Design review of the part built by this model. Coordinates are the model's own, in mm. Round coordinates to 2 decimals unless told otherwise and drop trailing zeros. Loops run counter-clockwise (first coordinate to the right, second up) from the corner with the lowest first, then second, coordinate; pieces in that order, holes last. Notation, with made-up numbers: (-32, -8.5) -> (-28, -8.5) arc R8 cw to (-28, -1.5) -> close; hole circle Ø11 at (89, 69). An arc over 180 degrees is marked (long way). Use a Markdown table: item, result. Add a question column.
from build123d import *

# Parameters (mm, degrees)
SKETCH1_R           = 3.9751
SKETCH1_R_2         = 6.35
BOSS_EXTRUDE1_DEPTH = 3.175


with BuildPart() as part:
    # Sketch1 → Boss-Extrude1 (new body)
    with BuildSketch(Plane.XY):
        with BuildLine():
            Line((-25.4, 88.9), (25.4, 88.9))
            Line((25.4, 88.9), (50.793088675, 18.258224664))
            ThreePointArc((50.793088675, 18.258224664), (0, -53.975), (-50.793088675, 18.258224664))
            Line((-50.793088675, 18.258224664), (-25.4, 88.9))
        make_face()
        with Locations((14.2875, 79.375)):
            Circle(SKETCH1_R, mode=Mode.SUBTRACT)
        with Locations(Location((-14.2875, 79.375, 0), (0, 0, 180))):
            Circle(SKETCH1_R, mode=Mode.SUBTRACT)
        Circle(SKETCH1_R_2, mode=Mode.SUBTRACT)
    extrude(amount=BOSS_EXTRUDE1_DEPTH)


solid = part.part
1. Insertion check: P1, Ø1, axis at y = 37, z = 2, coming from the +X side; P2, Ø6.5, axis at x = -14.29, y = 79.38, coming from the +Z side. Each pin has a flat end and moves straight along its axis. Give the tip position at first contact, or say it passes through.
2. To check wall thickness, follow probe 1 along X at (y, z) = (83, 1.4); probe 2 along Y at (x, z) = (3, 0.35); probe 3 along Y at (x, z) = (2, 1.05). State the ranges of each line that lie inside material, in increasing order. Write a range as from..to.
3. Consider section D-D on y = 23.5. State the section outline as (x, z) points (3 decimals).
4. Mouldability with a two-part tool opening along X and no side actions: class faces 1 (the face through (-1.38, -6.2, 1.57)), 2 (the face through (37.92, 54.07, 1.57)), 3 (the face through (1.448, -53.956, 1.565)) as +X half, -X half, draft (parallel to the pull), parting line (faces both ways), or undercut.
5. Consider section C-C on z = 2.4. Give the number of separate pieces and of enclosed holes in the cut face, plus the area to 3 significant figures.
6. Consider section A-A on x = 16.5. State the section outline as (y, z) points (3 decimals), plus the area to 3 significant figures.
7. Consider section B-B on y = 0. State the section outline as (x, z) points (3 decimals), plus the area to 3 significant figures.
Verdict:
| question | item | result |
|---|---|---|
| 1 | P1 | stops at x = 44.24 |
| 1 | P2 | passes through |
| 2 | probe 1 | x = -27.52..-15.92, -12.66..12.66, 15.92..27.52 |
| 2 | probe 2 | y = -53.89..-5.6, 5.6..88.9 |
| 2 | probe 3 | y = -53.94..-6.03, 6.03..88.9 |
| 3 | outline | (-48.909, 0) -> (48.909, 0) -> (48.909, 3.175) -> (-48.909, 3.175) -> close |
| 4 | face 1 | undercut |
| 4 | face 2 | +X half |
| 4 | face 3 | parting line |
| 5 | separate pieces | 1 |
| 5 | enclosed holes | 3 |
| 5 | area | 11,700 mm² |
| 6 | outline | (-51.391, 0) -> (76.073, 0) -> (76.073, 3.175) -> (-51.391, 3.175) -> close; (82.677, 0) -> (88.9, 0) -> (88.9, 3.175) -> (82.677, 3.175) -> close |
| 6 | area | 424 mm² |
| 7 | outline | (-53.975, 0) -> (-6.35, 0) -> (-6.35, 3.175) -> (-53.975, 3.175) -> close; (6.35, 0) -> (53.975, 0) -> (53.975, 3.175) -> (6.35, 3.175) -> close |
| 7 | area | 302 mm² |
